Verification items for this drawing (mm, ordinates from the low corner). A direction names the side the tool comes from. Round coordinates to 2 decimals unless told otherwise and drop trailing zeros. Order: outer loops, then holes, each group sorted by start corner. A loop starts at its lowest first (then second) coordinate and runs counter-clockwise, first axis right, second up. Notation, with made-up numbers: M -27,-23.75 L 25,-23.75 A22 ccw 25,-15.75 Z; hole C -29,-3.75 d6. An arc over 180 degrees is marked long. One line per item, written item: value. Start each with the question number.
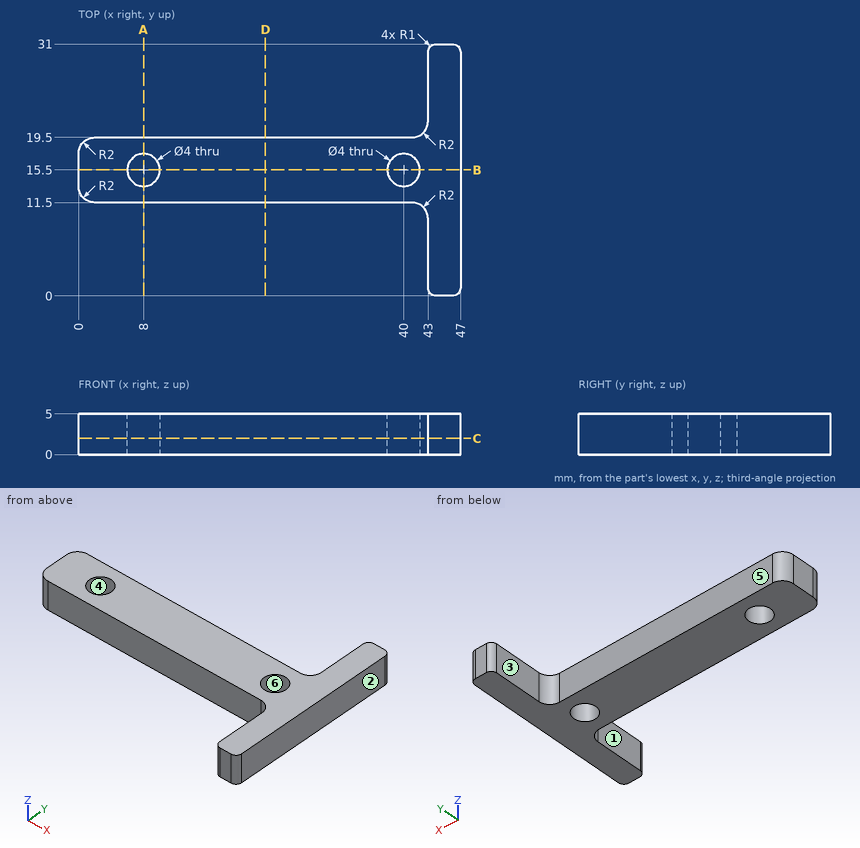
1. Section check D-D (x = 23). Record the cut outline in (y, z).
2. Tool access check on the marked faces 1 and 2. Record the directions out of +Z, -Z, +X, -X, +Y, -Y that give a thin tool (end or side, any length) a straight path to the whole face; none if there is none.
3. Section check A-A (x = 8). Record the cut outline in (y, z), and give its area (3 significant figures).
4. Depth check by flat-ended pin: pin 1 (2.5 mm diameter, centred on x = 13, z = 2, fed in from -Y); pin 2 (1.5 mm diameter, centred on y = 26, z = 1.5, fed in from -X); pin 3 (8 mm diameter, centred on x = 33.5, y = 25, fed in from -Z); pin 4 (2 mm diameter, centred on x = 28.5, z = 1.5, fed in from +Y). Enter the tip coordinate at first touch or a pass-through.
5. Draft check along Y on the marked faces 3, 4, 5 and 6. Enter one of: released by +Y, released by -Y, zero draft, split by the parting line, or undercut.
6. Section check C-C (z = 2). Record the cut outline in (x, y).
7. Scan lines: line 1 along Y through (x, z) = (40, 3.2); line 2 along Y through (x, z) = (20.5, 1); line 3 along X through (y, z) = (14, 1.3). Record each from-to range of solid material in increasing order.
8. Section check B-B (y = 15.5). Record the cut outline in (x, z), and give its area (3 significant figures).
Geometry check:
1. outline: M 11.5,0 L 19.5,0 L 19.5,5 L 11.5,5 Z
2. face 1: +Z, -Z, -X, -Y
2. face 2: +Z, -Z, +X, +Y, -Y
3. outline: M 11.5,0 L 13.5,0 L 13.5,5 L 11.5,5 Z; M 17.5,0 L 19.5,0 L 19.5,5 L 17.5,5 Z
3. area: 20.0 mm²
4. pin 1: stops at y = 11.5
4. pin 2: stops at x = 43
4. pin 3: passes through
4. pin 4: stops at y = 19.5
5. face 3: zero draft
5. face 4: undercut
5. face 5: released by +Y
5. face 6: undercut
6. outline: M 0,13.5 A2 ccw 2,11.5 L 41,11.5 A2 cw 43,9.5 L 43,1 A1 ccw 44,0 L 46,0 A1 ccw 47,1 L 47,30 A1 ccw 46,31 L 44,31 A1 ccw 43,30 L 43,21.5 A2 cw 41,19.5 L 2,19.5 A2 ccw 0,17.5 Z; hole C 8,15.5 d4; hole C 40,15.5 d4
7. line 1: y = 11.5 to 13.5, 17.5 to 19.5
7. line 2: y = 11.5 to 19.5
7. line 3: x = 0 to 6.68, 9.32 to 38.68, 41.32 to 47
8. outline: M 0,0 L 6,0 L 6,5 L 0,5 Z; M 10,0 L 38,0 L 38,5 L 10,5 Z; M 42,0 L 47,0 L 47,5 L 42,5 Z
8. area: 195 mm²
